Source: three-view drawing plus pictorial views. Frame: mm from the lowest corner of the part. A direction names the side the tool comes from. Give positions to 0.01 mm unless a question says otherwise; leave off trailing zeros. Write each loop counter-clockwise with the first axis right and the second up, starting at its lowest first coordinate (ties: lowest second). Pieces come first, ordered by that corner, then holes. Notation, with made-up numbers: (30, 40) -> (65, 40) arc R19 cw to (65, 71) -> close; hole circle Ø3 at (23.5, 42). An arc over 180 degrees is marked (long way). Answer in a Markdown table with one row per item. Add a question column.
Item 1: Access query for the marked faces 1 and 2. Directions: +Z, -Z, +X, -X, +Y, -Y. A direction counts if a zero-diameter tool reaches every point of the face in a straight line with its end or side. Return the directions, or none.
Item 2: First-contact query: P1, Ø1.5, axis at x = 16, y = 8, coming from the +Z side. Flat tip, straight axial feed; report the tip coordinate or a pass-through.
Item 3: Draft query along Y for the marked faces 3, 4, 5 and 6. Return one class per face: +Y half, -Y half, draft (parallel to the pull), parting line (faces both ways), or undercut.
Item 4: Section query B-B on y = 25.5. Output: boundary loops of the cut face in (x, z) (1 decimal).
Item 5: Section query A-A on y = 5. Output: boundary loops of the cut face in (x, z) (1 decimal).
Item 6: Section query D-D on z = 2.25. Output: boundary loops of the cut face in (x, y), plus the area to 3 significant figures.
Item 7: Material intervals for probe 1 along Y at (x, z) = (26.5, 5.75); probe 2 along Y at (x, z) = (28, 4) (1 decimal); probe 3 along X at (y, z) = (26.5, 11.5) (1 decimal), sorted ascending. Write a range as from..to.
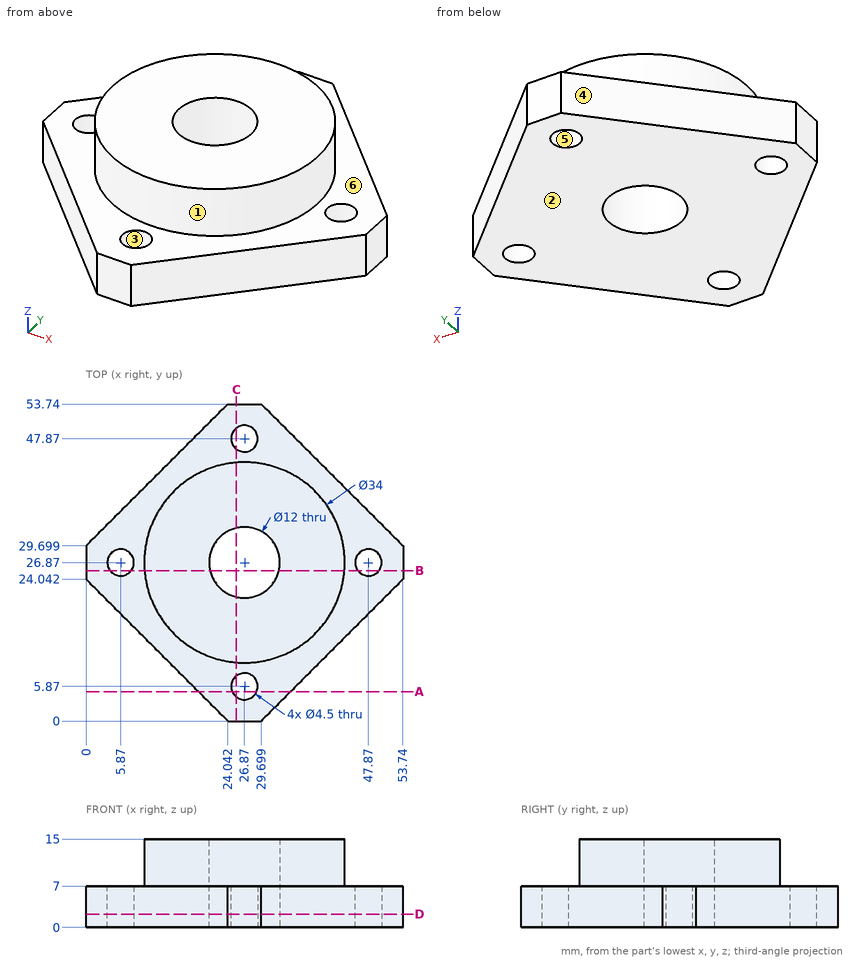
Findings below:
| question | item | result |
|---|---|---|
| 1 | face 1 | +Z |
| 1 | face 2 | -Z, +X, -X, +Y, -Y |
| 2 | P1 | stops at z = 7 |
| 3 | face 3 | undercut |
| 3 | face 4 | +Y half |
| 3 | face 5 | undercut |
| 3 | face 6 | draft |
| 4 | outline | (0, 0) -> (4.1, 0) -> (4.1, 7) -> (0, 7) -> close; (7.7, 0) -> (21, 0) -> (21, 15) -> (9.9, 15) -> (9.9, 7) -> (7.7, 7) -> close; (32.7, 0) -> (46.1, 0) -> (46.1, 7) -> (43.8, 7) -> (43.8, 15) -> (32.7, 15) -> close; (49.7, 0) -> (53.7, 0) -> (53.7, 7) -> (49.7, 7) -> close |
| 5 | outline | (19, 0) -> (24.8, 0) -> (24.8, 7) -> (19, 7) -> close; (28.9, 0) -> (34.7, 0) -> (34.7, 7) -> (28.9, 7) -> close |
| 6 | outline | (0, 24.04) -> (24.04, 0) -> (29.7, 0) -> (53.74, 24.04) -> (53.74, 29.7) -> (29.7, 53.74) -> (24.04, 53.74) -> (0, 29.7) -> close; hole circle Ø4.5 at (5.87, 26.87); hole circle Ø12 at (26.87, 26.87); hole circle Ø4.5 at (26.87, 5.87); hole circle Ø4.5 at (26.87, 47.87); hole circle Ø4.5 at (47.87, 26.87) |
| 6 | area | 1,560 mm^2 |
| 7 | probe 1 | y = 0..3.65, 8.09..20.88, 32.86..45.65, 50.09..53.74 |
| 7 | probe 2 | y = 0..3.9, 7.8..21, 32.8..45.9, 49.8..53.7 |
| 7 | probe 3 | x = 9.9..20.9, 32.9..43.9 |
